```python
from build123d import *

# Parameters (mm, degrees)
F1_DEPTH = 20
F2_R     = 3


with BuildPart() as f1:
    # F0 (on Front) → F1 (new body)
    with BuildSketch(Plane.XZ):
        with BuildLine():
            Line((8.25, 0), (4.25, 0))
            ThreePointArc((4.25, 0), (-3.00520382, -3.00520382), (0, 4.25))
            Line((0, 4.25), (0, 14))
            Line((0, 14), (-20, 14))
            Line((-20, 14), (-20, 0))
            Line((-20, 0), (-20, -14))
            Line((-20, -14), (0, -14))
            Line((0, -14), (8.25, -14))
            Line((8.25, -14), (8.25, 0))
        make_face()
        with BuildLine():
            ThreePointArc((0, 4.25), (3.00520382, 3.00520382), (4.25, 0))
            Line((4.25, 0), (8.25, 0))
            Line((8.25, 0), (0, 14))
            Line((0, 14), (0, 4.25))
        make_face()
    extrude(amount=-F1_DEPTH)

    # F2
    f2_edges = [f1.edges().sort_by_distance(p)[0] for p in [
        (0, 10, 14),
        (8.25, 10, 0),
        (-20, 10, 14),
        (-20, 20, 0),
        (-10, 0, 14),
        (-20, 0, 0),
        (-5.875, 0, -14),
        (8.25, 0, -7),
        (-10, 20, 14),
        (-5.875, 20, -14),
        (8.25, 10, -14),
        (8.25, 20, -7),
        (-20, 10, -14),
    ]]
    fillet(f2_edges, radius=F2_R)


solid = f1.part
```
The model under review builds one solid part; all positions refer to its coordinate system, in mm. Round coordinates to 2 decimals unless told otherwise and drop trailing zeros. Loops run counter-clockwise (first coordinate to the right, second up) from the corner with the lowest first, then second, coordinate; pieces in that order, holes last. Notation, with made-up numbers: (-34, 74.5) - (-24, 74.5) arc R21 ccw to (-24, 94.5) - close; hole circle Ø6 at (27, -15). An arc over 180 degrees is marked (long way). Write each question's results on one line, items separated by ' | '. Start each with the question number.
Q1. Take a section at D-D on y = 2.5. Give the boundary of the cut face in (x, z), plus the area to 3 significant figures.
Q2. Wall thickness on line 1 along X through (y, z) = (11, -1.25); line 2 along Z through (x, y) = (-1.75, 9.25); line 3 along X through (y, z) = (17, 2.25): over which ranges is each line inside the solid? List them lowest first. Write a range as [from, to].
Q3. Take a section at A-A on z = 3.75. Give the boundary of the cut face in (x, y).
Q4. Take a section at B-B on y = 10. Give the boundary of the cut face in (x, z), plus the area to 3 significant figures.
Q5. Take a section at C-C on x = -0.75. Give the boundary of the cut face in (y, z).
Q6. Insertion check: P1, Ø7.5, axis at x = 0, z = 0, coming from the +Y side; P2, Ø4, axis at y = 13, z = 10.5, coming from the +X side. Each pin has a flat end and moves straight along its axis. Give the tip position at first contact, or say it passes through.
Data:
1) outline: (-19.96, -11) arc R2.96 ccw to (-17, -13.96) - (5.25, -13.96) arc R2.96 ccw to (8.21, -11) - (8.21, -0.32) arc R3 ccw to (7.83, 0.7) - (0.87, 12.52) arc R3 ccw to (-1.21, 13.96) - (-17, 13.96) arc R2.96 ccw to (-19.96, 11) - close; hole circle Ø8.5 at (0, 0) | area: 667 mm²
2) line 1: x = [-20, -4.06], [4.06, 8.25] | line 2: z = [-14, -3.87], [3.87, 14] | line 3: x = [-20, -3.61], [3.61, 6.92]
3) outline: (-20, 3) arc R3 ccw to (-17, 0) - (-2, 0) - (-2, 20) - (-17, 20) arc R3 ccw to (-20, 17) - close; (2, 0) - (5.25, 0) arc R3 ccw to (6.04, 0.11) - (6.04, 19.89) arc R3 ccw to (5.25, 20) - (2, 20) - close
4) outline: (-20, -11) arc R3 ccw to (-17, -14) - (5.25, -14) arc R3 ccw to (8.25, -11) - (8.25, -0.82) arc R3 ccw to (7.83, 0.7) - (0.87, 12.52) arc R3 ccw to (-1.71, 14) - (-17, 14) arc R3 ccw to (-20, 11) - close; hole circle Ø8.5 at (0, 0) | area: 670 mm²
5) outline: (0, -11) arc R3 ccw to (3, -14) - (17, -14) arc R3 ccw to (20, -11) - (20, -4.18) - (0, -4.18) - close; (0, 4.18) - (20, 4.18) - (20, 11) arc R3 ccw to (17.96, 13.84) - (2.04, 13.84) arc R3 ccw to (0, 11) - close
6) P1: passes through | P2: stops at x = 3.24
